Could you check a few things on this drawing? It's one solid part, dimensions in mm from its lowest x, y, z. A direction names the side the tool comes from. Coordinates: 2 decimals unless noted, no trailing zeros. Write each loop counter-clockwise with the first axis right and the second up, starting at its lowest first coordinate (ties: lowest second). Pieces come first, ordered by that corner, then holes.
Item 1: I'm going to push flat-ended pins straight in: P1, Ø1.2, axis at y = 37.5, z = 1, coming from the +X side; P2, Ø0.8, axis at y = 38.5, z = 1, coming from the -X side; P3, Ø1.2, axis at x = 41.5, z = 1.5, coming from the +Y side. Where does each tip first touch, or does it pass through?
Item 2: I want a section at A-A (z = 10). Please give me the cut outline in (x, y).
Item 3: I want a section at C-C (x = 28.5). Please give me the cut outline in (y, z), and give its area (3 significant figures).
Item 4: For the marked faces 1 and 2, which set-ups out of +Z, -Z, +X, -X, +Y, -Y let a thin tool reach every point of the face, with its end or its side?
Item 5: Please list where these lines run through material, in increasing order: line 1 (Z direction, x = 32, y = 41); line 2 (X direction, y = 33.5, z = 1.25).
Item 6: I want a section at D-D (y = 32). Please give me the cut outline in (x, z).
Item 7: I want a section at B-B (y = 39). Please give me the cut outline in (x, z), and give its area (3 significant figures).
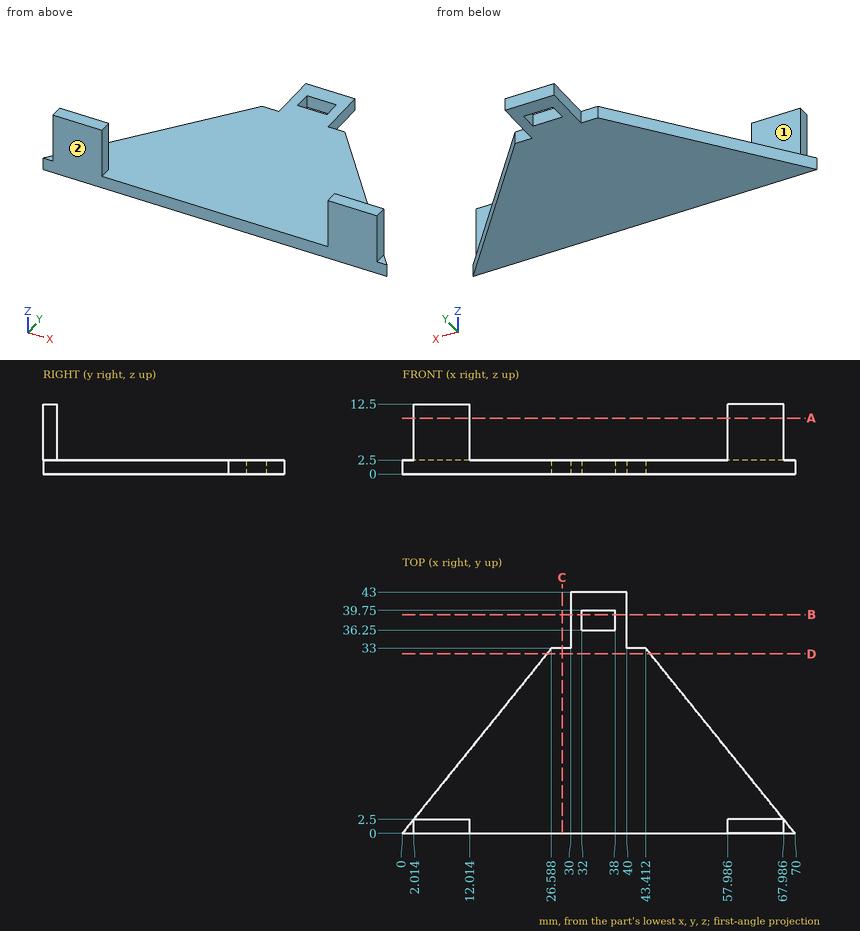
Answer:
1. P1: stops at x = 40
1. P2: stops at x = 30
1. P3: stops at y = 33
2. outline: (2.01, 0) - (12.01, 0) - (12.01, 2.5) - (2.01, 2.5) - close; (57.99, 0) - (67.99, 0) - (67.99, 2.5) - (57.99, 2.5) - close
3. outline: (0, 0) - (33, 0) - (33, 2.5) - (0, 2.5) - close
3. area: 82.5 mm2
4. face 1: +Z, +X, -X, +Y
4. face 2: +Z, -Z, +X, -X, -Y
5. line 1: z = 0 to 2.5
5. line 2: x = 30 to 40
6. outline: (25.78, 0) - (44.22, 0) - (44.22, 2.5) - (25.78, 2.5) - close
7. outline: (30, 0) - (32, 0) - (32, 2.5) - (30, 2.5) - close; (38, 0) - (40, 0) - (40, 2.5) - (38, 2.5) - close
7. area: 10.0 mm2
